Input: part model. Units: mm. Frame: model coordinates. Coordinates: 2 decimals unless noted, no trailing zeros. Write each loop counter-clockwise with the first axis right and the second up, starting at its lowest first coordinate (ties: lowest second). Pieces come first, ordered by that corner, then holes. Notation, with made-up numbers: M 58,83.25 L 102,83.25 A8 cw 102,98.25 Z; hole C 69,43 d8. An arc over 180 degrees is marked long. Use one line per item in the form item = value.
from build123d import *

# Parameters (mm, degrees)
SKETCH_1_R           = 50
SKETCH_1_R_2         = 40
EXTRUDE_1_DEPTH      = 50
EXTRUDE_2_REACH      = 238.422
EXTRUDE_2_END_RADIUS = 50
SKETCH_2_R           = 30


with BuildPart() as part:
    # 草图1 → 凸台-拉伸1 (new, symmetric)
    with BuildSketch(Plane(origin=(0, 0, 0), x_dir=(0, 0, -1), z_dir=(1, 0, 0))):
        Circle(SKETCH_1_R)
        Circle(SKETCH_1_R_2, mode=Mode.SUBTRACT)
    extrude_1 = extrude(amount=EXTRUDE_1_DEPTH, both=True)

    # 凸台-拉伸2: up to this cylinder (the profile starts outside it)
    extrude_2_end = Plane(origin=(0, 0, 0), z_dir=(1, 0, 0)) * Cylinder(EXTRUDE_2_END_RADIUS, 577.844, mode=Mode.PRIVATE)
    # 草图2 → 凸台-拉伸2 (add, up to the surface)
    with BuildSketch(Plane(origin=(0, -175.6, 0), x_dir=(1, 0, 0), z_dir=(0, 1, 0)), mode=Mode.PRIVATE) as extrude_2_sk1:
        with Locations(Location((0, 0, 0), (0, 0, 90))):
            Circle(SKETCH_2_R)
    extrude_2_tool1 = extrude(extrude_2_sk1.sketch, amount=EXTRUDE_2_REACH, mode=Mode.PRIVATE) - extrude_2_end
    extrude_2 = extrude_2_tool1.solids().sort_by_distance((0, -175.6, 0))[0]
    add(extrude_2)

    # 镜向4: 凸台-拉伸2 across plane
    add(extrude_2.mirror(Plane.ZX.offset(-175.6)))

    # 镜向5: 凸台-拉伸1 across plane
    add(extrude_1.mirror(Plane.ZX.offset(-175.6)))


solid = part.part
(1) Section query A-A on z = 0. Return the cut outline in (x, y), plus the area to 3 significant figures.
Computed:
outline = M -50,-401.2 L 50,-401.2 L 50,-391.2 L -50,-391.2 Z; M -50,-311.2 L 50,-311.2 L 50,-301.2 L 30,-301.2 L 30,-50 L 50,-50 L 50,-40 L -50,-40 L -50,-50 L -30,-50 L -30,-301.2 L -50,-301.2 Z; M -50,40 L 50,40 L 50,50 L -50,50 Z
area = 19,100 mm^2
(2) Section query B-B on y = -351.2. Return the cut outline in (x, z).
Computed:
outline = M -50,-50 L 50,-50 L 50,-40 L -50,-40 Z; M -50,40 L 50,40 L 50,50 L -50,50 Z
(3) Section query C-C on x = 0. Return the cut outline in (y, z).
Computed:
outline = M -311.2,-30 L -40,-30 A50 ccw long -40,30 L -311.2,30 A50 ccw long Z; hole C -351.2,0 d80; hole C 0,0 d80
(4) First-contact query: pin 1 Ø1 at (y, z) = (-290, 8) entering from -X; pin 2 Ø3 at (y, z) = (-288, 12) entering from +X; pin 3 Ø1.5 at (x, y) = (-6, -335.5) entering from -Z; pin 4 Ø1.5 at (x, y) = (-31.5, -71) entering from -Z. Flat tips, straight axial feed; report the tip coordinate or a pass-through.
Computed:
pin_1 = -29.05
pin_2 = 28.1
pin_3 = -47.71
pin_4 = through
(5) Pull-direction query (Y, two-part tool) for faces 1 (the cylindrical face through (0.7, 49.575, 6.509)), 2 (the flat face through (50, 34, 22)); classes: pulls with the +Y half, pulls with the -Y half, needs draft (parallel to the pull), parting line crosses it, or undercut.
Computed:
face_1 = undercut
face_2 = needs draft
(6) Section query D-D on x = 39. Return the cut outline in (y, z).
Computed:
outline = C -351.2,0 d100; C 0,0 d100; hole C -351.2,0 d80; hole C 0,0 d80
(7) Line query: probe 1 along Y at (x, z) = (-7, 0); probe 2 along Z at (x, y) = (9.5, -351.2); probe 3 along Y at (x, z) = (-40, -28). Output: solid intervals per line, ascending.
Computed:
probe_1 = -401.2 to -391.2, -311.2 to -40, 40 to 50
probe_2 = -50 to -40, 40 to 50
probe_3 = -392.62 to -379.77, -322.63 to -309.78, -41.42 to -28.57, 28.57 to 41.42
